from build123d import *

# Parameters (mm, degrees)
SKETCH1_W           = 60.566280351
SKETCH1_H           = 41.91
BOSS_EXTRUDE1_DEPTH = 2
BOSS_EXTRUDE2_DEPTH = 60.56628035
CUT_EXTRUDE1_REACH  = 54.849
SKETCH5_R           = 1.5
SKETCH6_R           = 2.7
CUT_EXTRUDE2_DEPTH  = 4.1
SKETCH9_R           = 2.7
CUT_EXTRUDE3_DEPTH  = 4.1


with BuildPart() as part:
    # Sketch1 → Boss-Extrude1 (new body)
    with BuildSketch(Plane(origin=(0, 0, 0), x_dir=(1, 0, 0), z_dir=(0, 1, 0))):
        with Locations((0.392342893, 1.258772873)):
            Rectangle(SKETCH1_W, SKETCH1_H)
    extrude(amount=BOSS_EXTRUDE1_DEPTH)

    # Sketch4 → Boss-Extrude2 (add)
    with BuildSketch(Plane.ZY.offset(29.890797283)):
        with BuildLine():
            Line((-22.21383483, 1.959789744), (-9.274266868, 1.959789744))
            Line((-9.274266868, 1.959789744), (-11.775730551, 4.430225514))
            ThreePointArc((-11.775730551, 4.430225514), (-11.903861669, 4.791947782), (-11.793775933, 5.15956404))
            Line((-11.793775933, 5.15956404), (-9.222914706, 7.723241684))
            Line((-9.222914706, 7.723241684), (-9.232672854, 9.668426415))
            Line((-9.232672854, 9.668426415), (-22.252178068, 9.603113205))
            Line((-22.252178068, 9.603113205), (-22.21383483, 1.959789744))
        make_face()
        with BuildLine():
            Line((6.756821981, 2), (19.696227127, 2))
            Line((19.696227127, 2), (19.696227127, 9.708331019))
            Line((19.696227127, 9.708331019), (6.676558091, 9.708331019))
            Line((6.676558091, 9.708331019), (6.676558091, 7.763121812))
            Line((6.676558091, 7.763121812), (9.260247666, 5.212373159))
            ThreePointArc((9.260247666, 5.212373159), (9.372176165, 4.845313772), (9.24586124, 4.482953285))
            Line((9.24586124, 4.482953285), (6.756821981, 2))
        make_face()
    extrude(amount=-BOSS_EXTRUDE2_DEPTH)

    # Cut-Extrude1: up to this plane
    cut_extrude1_end = Plane(origin=(-29.890797283, 2, 19.696227127), z_dir=(0, 0, -1))
    # Sketch5 → Cut-Extrude1 (cut, up to the surface)
    with BuildSketch(Plane(origin=(0, -0.111385049, -22.203444644), x_dir=(-1, 0, 0), z_dir=(0, -0.005016503049651579, -0.9999874172694139)), mode=Mode.PRIVATE) as cut_extrude1_sk1:
        with Locations(Location((14.607657107, 5.892910673, 0), (0, 0, 331.006868197))):
            Circle(SKETCH5_R)
    cut_extrude1_tool1 = split(extrude(cut_extrude1_sk1.sketch, amount=-CUT_EXTRUDE1_REACH, mode=Mode.PRIVATE), bisect_by=cut_extrude1_end, keep=Keep.BOTH, mode=Mode.PRIVATE)
    add(cut_extrude1_tool1.solids().sort_by_distance((-14.607657, 5.781451, -22.233006))[0], mode=Mode.SUBTRACT)
    # Sketch5 → Cut-Extrude1 (cut, up to the surface)
    with BuildSketch(Plane(origin=(0, -0.111385049, -22.203444644), x_dir=(-1, 0, 0), z_dir=(0, -0.005016503049651579, -0.9999874172694139)), mode=Mode.PRIVATE) as cut_extrude1_sk2:
        with Locations(Location((-15.392342893, 5.892910673, 0), (0, 0, 331.006868197))):
            Circle(SKETCH5_R)
    cut_extrude1_tool2 = split(extrude(cut_extrude1_sk2.sketch, amount=-CUT_EXTRUDE1_REACH, mode=Mode.PRIVATE), bisect_by=cut_extrude1_end, keep=Keep.BOTH, mode=Mode.PRIVATE)
    add(cut_extrude1_tool2.solids().sort_by_distance((15.392343, 5.781451, -22.233006))[0], mode=Mode.SUBTRACT)

    # Sketch6 → Cut-Extrude2 (cut)
    with BuildSketch(Plane(origin=(0, -0.111385049, -22.203444644), x_dir=(-1, 0, 0), z_dir=(0, -0.005016503049651579, -0.9999874172694139))):
        with Locations(Location((14.607657107, 5.892910673, 0), (0, 0, 90))):
            Circle(SKETCH6_R)
        with Locations(Location((-15.392342893, 5.892910673, 0), (0, 0, 90))):
            Circle(SKETCH6_R)
    extrude(amount=-CUT_EXTRUDE2_DEPTH, mode=Mode.SUBTRACT)

    # Sketch9 → Cut-Extrude3 (cut)
    with BuildSketch(Plane.XY.offset(19.696227127)):
        with Locations((15.392342893, 5.991792249)):
            Circle(SKETCH9_R)
        with Locations((-14.607657107, 5.991792249)):
            Circle(SKETCH9_R)
    extrude(amount=-CUT_EXTRUDE3_DEPTH, mode=Mode.SUBTRACT)


solid = part.part
Geometry check sheet. Reference: the model listing, model coordinates, mm. A direction names the side the tool comes from. Round coordinates to 2 decimals unless told otherwise and drop trailing zeros. Write each loop counter-clockwise with the first axis right and the second up, starting at its lowest first coordinate (ties: lowest second). Pieces come first, ordered by that corner, then holes.
Item 1: Section check C-C (y = 6.75). Give the number of separate pieces and of enclosed holes in the cut face, plus the area to 3 significant figures.
Determined:
separate pieces: 6
enclosed holes: 0
area: 1,290 mm2
Item 2: Section check B-B (z = 4). Record the boundary of the cut face in (x, y), plus the area to 3 significant figures.
Determined:
outline: (-29.89, 0) - (30.68, 0) - (30.68, 2) - (-29.89, 2) - close
area: 121 mm2
Item 3: Access from +Z, -Z, +X, -X, +Y, -Y to the whole of each face (thin tool, end or side, straight path). Record for faces 1 (the face through (-0.03, 3.2, -10.53)), 2 (the face through (-12.03, 6.8, 17.67)).
Determined:
face 1: +X, -X
face 2: +Z
Item 4: Material ranges on line 1 along Z through (x, y) = (0, 7.75); line 2 along X through (y, z) = (7, -11); line 3 along Y through (x, z) = (-7, 1.5), recorded low to high.
Determined:
line 1: z = -22.24 to -9.22, 6.69 to 19.7
line 2: x = -29.89 to -15.56, -13.66 to 14.44, 16.34 to 30.68
line 3: y = 0 to 2
Item 5: Go/stop test with flat-tipped pins: pin 1 Ø1.5 at (x, y) = (-15, 1.5) entering from -Z; pin 2 Ø1.5 at (x, z) = (20.5, -3) entering from -Y; pin 3 Ø2.5 at (x, y) = (-15.5, 5) entering from +Z; pin 4 Ø13 at (x, z) = (15, -3.5) entering from +Y. Record where each tip stops, or that it passes through.
Determined:
pin 1: stops at z = -22.22
pin 2: stops at y = 0
pin 3: stops at z = 15.6
pin 4: stops at y = 9.67
Item 6: Mould release check, pull along Z, two halves, no side actions. Record for faces 3 (the face through (17, 5, 15.596)), 4 (the face through (0, 2, -1)), 5 (the face through (17.97, 6.8, 17.67)): +Z half, -Z half, draft (parallel to the pull), parting line (faces both ways), or undercut.
Determined:
face 3: +Z half
face 4: undercut
face 5: draft
